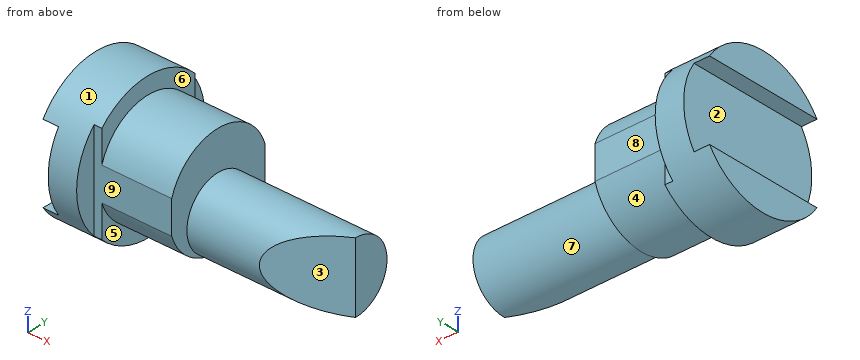
```python
from build123d import *

# Parameters (mm, degrees)
F2_R     = 13.5
F3_DEPTH = 53
F5_DEPTH = 30
F6_W     = 6
F6_H     = 30
F7_DEPTH = 27.5
F9_DEPTH = 25


# Not quite as in the source:
# - a feature names something its author has since deleted; it is built from what else it names


with BuildPart() as f1:
    # F0 (on Front) → F1 (revolve)
    with BuildSketch(Plane.XZ):
        Polygon((0, 27.5), (0, 0), (47, 0), (47, 21), (20, 21), (20, 27.5), align=None)
    revolve(axis=Axis((37.6517102122, 0, 0), (1, 0, 0)))

    # F2 (on face) → F3 (join)
    with BuildSketch(Plane.YZ.offset(47)):
        with Locations((0, -7.5)):
            Circle(F2_R)
    extrude(amount=F3_DEPTH)

    # F4 (on face) → F5 (cut)
    with BuildSketch(Plane.YZ.offset(47)):
        with BuildLine():
            ThreePointArc((20, -18.8745860882), (25.5563103753, -10.1550480058), (27.5, 0))
            ThreePointArc((27.5, 0), (25.5563103753, 10.1550480058), (20, 18.8745860882))
            Line((20, 18.8745860882), (20, 6.4031242374))
            ThreePointArc((20, 6.4031242374), (21, 0), (20, -6.4031242374))
            Line((20, -6.4031242374), (20, -18.8745860882))
        make_face()
        with BuildLine():
            Line((-20, 6.4031242374), (-20, 18.8745860882))
            ThreePointArc((-20, 18.8745860882), (-27.5, 0), (-20, -18.8745860882))
            Line((-20, -18.8745860882), (-20, -6.4031242374))
            ThreePointArc((-20, -6.4031242374), (-21, 0), (-20, 6.4031242374))
        make_face()
        with BuildLine():
            ThreePointArc((20, -6.4031242374), (21, 0), (20, 6.4031242374))
            Line((20, 6.4031242374), (20, -6.4031242374))
        make_face()
        with BuildLine():
            Line((-20, -6.4031242374), (-20, 6.4031242374))
            ThreePointArc((-20, 6.4031242374), (-21, 0), (-20, -6.4031242374))
        make_face()
    extrude(amount=-F5_DEPTH, mode=Mode.SUBTRACT)

    # F6 (on Front) → F7 (cut, symmetric)
    with BuildSketch(Plane.XZ):
        with Locations((3, 0)):
            Rectangle(F6_W, F6_H)
    extrude(amount=F7_DEPTH, both=True, mode=Mode.SUBTRACT)

    # F8 (on Top) → F9 (cut, symmetric)
    with BuildSketch(Plane.XY):
        Polygon((100, -13.5), (100, 0), (75, -13.5), align=None)
    extrude(amount=F9_DEPTH, both=True, mode=Mode.SUBTRACT)


solid = f1.part
```
Geometry check sheet. Reference: the model listing, model coordinates, mm. Face numbers are marked on the shaded views. A direction names the side the tool comes from. Coordinates: 2 decimals unless noted, no trailing zeros. Order: outer loops, then holes, each group sorted by start corner. A loop starts at its lowest first (then second) coordinate and runs counter-clockwise, first axis right, second up. Notation, with made-up numbers: (42, 22) - (93, 22) arc R30 ccw to (93, 50) - close; hole circle Ø5 at (34, -27). An arc over 180 degrees is marked (long way). Answer as a JSON object with one key per item and string values. Group by question number.
Item 1: Draft check along Z on the marked faces 1, 2, 3 and 4. Enter one of: +Z half, -Z half, draft (parallel to the pull), parting line (faces both ways), or undercut.
Item 2: Tool access check on the marked faces 5, 6, 7, 8 and 9. Record the directions out of +Z, -Z, +X, -X, +Y, -Y that give a thin tool (end or side, any length) a straight path to the whole face; none if there is none.
Item 3: Scan lines: probe 1 along X at (y, z) = (6.5, -14); probe 2 along X at (y, z) = (-17.5, 13); probe 3 along Z at (x, y) = (14.5, -7). Record each from-to range of solid material in increasing order.
Item 4: Sectioned sample at A-A, the plane z = -7.5. Record the cut outline in (x, y).
Item 5: Depth check by flat-ended pin: pin 1 Ø5 at (x, y) = (2.5, -1) entering from +Z; pin 2 Ø1.5 at (x, y) = (23, -16.5) entering from -Z; pin 3 Ø1.5 at (x, y) = (83, 1.5) entering from +Z; pin 4 Ø10 at (x, y) = (39, 6.5) entering from +Z. Enter the tip coordinate at first touch or a pass-through.
Item 6: Sectioned sample at C-C, the plane x = 71. Record the cut outline in (y, z), and give its area (3 significant figures).
Item 7: Sectioned sample at D-D, the plane z = 0. Record the cut outline in (x, y).
Item 8: Sectioned sample at B-B, the plane y = 16. Record the cut outline in (x, z).
Resolved:
{
 "1": {"face 1": "parting line", "face 2": "undercut", "face 3": "draft", "face 4": "-Z half"},
 "2": {"face 5": "-Z, +X", "face 6": "+Z, +X", "face 7": "+X", "face 8": "+Z, -Z, +X, +Y", "face 9": "+Z, -Z, +X, -Y"},
 "3": {"probe 1": "6 to 100", "probe 2": "6 to 20", "probe 3": "-26.59 to 26.59"},
 "4": {"outline": "(6, -26.46) - (17, -26.46) - (17, -20) - (20, -20) - (20, -19.62) - (47, -19.62) - (47, -13.5) - (75, -13.5) - (100, 0) - (100, 13.5) - (47, 13.5) - (47, 19.62) - (20, 19.62) - (20, 20) - (17, 20) - (17, 26.46) - (6, 26.46) - close"},
 "5": {"pin 1": "z = 27.5", "pin 2": "z = -13.89", "pin 3": "z = 5.98", "pin 4": "z = 20.95"},
 "6": {"outline": "circle Ø27 at (0, -7.5)", "area": "573 mm^2"},
 "7": {"outline": "(6, -27.5) - (17, -27.5) - (17, -20) - (47, -20) - (47, -11.22) - (79.21, -11.22) - (100, 0) - (100, 11.22) - (47, 11.22) - (47, 20) - (17, 20) - (17, 27.5) - (6, 27.5) - close"},
 "8": {"outline": "(0, -22.37) - (20, -22.37) - (20, -13.6) - (47, -13.6) - (47, 13.6) - (20, 13.6) - (20, 22.37) - (0, 22.37) - (0, 15) - (6, 15) - (6, -15) - (0, -15) - close"}
}
